Design review of the part built by this model. Coordinates are the model's own, in mm. Face numbers are marked on the shaded views. A direction names the side the tool comes from. Round coordinates to 2 decimals unless told otherwise and drop trailing zeros. Order: outer loops, then holes, each group sorted by start corner. A loop starts at its lowest first (then second) coordinate and runs counter-clockwise, first axis right, second up. Notation, with made-up numbers: M 13,82 L 28,82 A18 ccw 28,92 Z; hole C 13,42 d9. An arc over 180 degrees is marked long. Write each question's results on one line, items separated by ' | '. Start each with the question number.
Item 1: Take a section at C-C, the plane y = -16. Write out the cut boundary in (x, z).
Item 2: Clearance check with flat-ended pins moving along their axes: pin 1 (4 mm diameter, centred on x = 100, z = 2.5, fed in from +Y); pin 2 (1.9 mm diameter, centred on y = -26.5, z = 5.5, fed in from -X); pin 3 (5 mm diameter, centred on x = 10, y = -42, fed in from -Z); pin 4 (1.5 mm diameter, centred on x = 132, z = 11.5, fed in from -Y). State where each tip first meets the part, or that it passes through.
Item 3: Wall thickness on line 1 (Y direction, x = 50, z = 5.75); line 2 (Y direction, x = 124, z = 6.5); line 3 (Y direction, x = 124, z = 2.25): over which ranges is each line inside the solid? List them lowest first. Write a range as [from, to].
Item 4: Take a section at D-D, the plane x = 126.5. Write out the cut boundary in (y, z).
Item 5: Take a section at A-A, the plane x = 17. Write out the cut boundary in (y, z), plus the area to 3 significant figures.
Item 6: Take a section at B-B, the plane y = -25. Write out the cut boundary in (x, z), plus the area to 3 significant figures.
Item 7: Machinability: for the marked faces 1, 2 and 3, which of the approach directions +Z, -Z, +X, -X, +Y, -Y give a long, thin tool a straight path to every point of the face, cutting with its end or side? Answer none if there is none.
Item 8: The part is to be moulded in two halves that separate along Y. For the marked faces 4, 5 and 6, say which applies: +Y half, -Y half, draft (parallel to the pull), parting line (faces both ways), or undercut.
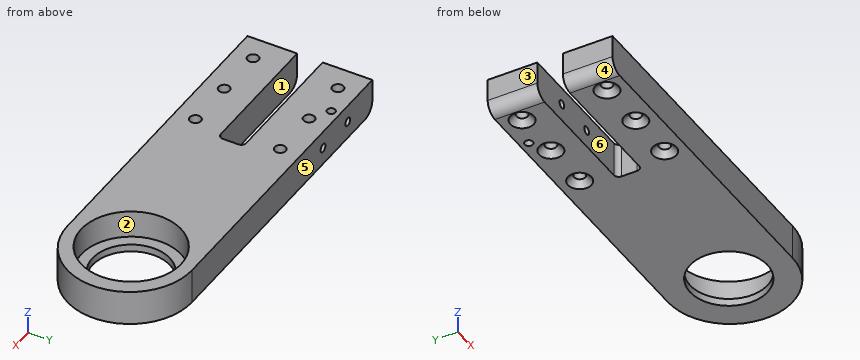
```python
from build123d import *

# Parameters (mm, degrees)
BOSS_EXTRUDE1_DEPTH       = 14
SKETCH2_W                 = 55
SKETCH2_H                 = 10.2
CUT_EXTRUDE1_DEPTH        = 15
F_8_CLEARANCE_HOLE1_D     = 4.5
F_8_CLEARANCE_HOLE1_DEPTH = 14
F_4_CLEARANCE_HOLE1_D     = 3.3
F_4_CLEARANCE_HOLE1_DEPTH = 14
F_4_CLEARANCE_HOLE2_D     = 3.3
F_4_CLEARANCE_HOLE2_DEPTH = 19.899999999
HOLE1_D                   = 31.000000009
HOLE1_DEPTH               = 14
HOLE1_CBORE_D             = 40.00000001
HOLE1_CBORE_DEPTH         = 11
CHAMFER1_SIZE             = 2.45
FILLET1_R                 = 2
FILLET2_R                 = 5


with BuildPart() as part:
    # Sketch1 → Boss-Extrude1 (new body)
    with BuildSketch(Plane(origin=(0, 0, 0), x_dir=(-1, 0, 0), z_dir=(0, 0, -1))):
        with BuildLine():
            Line((-125, -50), (0, -50))
            Line((0, -50), (0, 0))
            Line((0, 0), (-125, 0))
            ThreePointArc((-125, 0), (-150, -25), (-125, -50))
        make_face()
    extrude(amount=-BOSS_EXTRUDE1_DEPTH)

    # Sketch2 → Cut-Extrude1 (cut, through all)
    with BuildSketch(Plane.XY.offset(14)):
        with Locations((27.5, -24.999999999)):
            Rectangle(SKETCH2_W, SKETCH2_H)
    extrude(amount=-CUT_EXTRUDE1_DEPTH, mode=Mode.SUBTRACT)

    # #8 Clearance Hole1
    with Locations(Plane(origin=(0, 0, 0), x_dir=(-1, 0, 0), z_dir=(0, 0, -1))):
        with Locations((-10, -8), (-10, -42), (-30, -42), (-30, -8), (-50, -8), (-50, -42)):
            Hole(F_8_CLEARANCE_HOLE1_D / 2, depth=F_8_CLEARANCE_HOLE1_DEPTH)

    # #4 Clearance Hole1
    with Locations(Plane.XY.offset(14)):
        with Locations((22.5, -3.5)):
            Hole(F_4_CLEARANCE_HOLE1_D / 2, depth=F_4_CLEARANCE_HOLE1_DEPTH)

    # #4 Clearance Hole2
    with Locations(Plane(origin=(0, 0, 0), x_dir=(1, 0, 0), z_dir=(0, 1, 0))):
        with Locations((17, -7), (34.2, -7)):
            Hole(F_4_CLEARANCE_HOLE2_D / 2, depth=F_4_CLEARANCE_HOLE2_DEPTH)

    # Hole1
    with Locations(Plane.XY.offset(14)):
        with Locations((123.999999995, -24.999999999)):
            CounterBoreHole(HOLE1_D / 2, HOLE1_CBORE_D / 2, HOLE1_CBORE_DEPTH, depth=HOLE1_DEPTH)

    # Chamfer1
    chamfer1_edges = [part.edges().sort_by_distance(p)[0] for p in [
        (47.75, -42, 0),
        (47.75, -8, 0),
        (27.75, -8, 0),
        (27.75, -42, 0),
        (7.75, -42, 0),
        (7.75, -8, 0),
    ]]
    chamfer(chamfer1_edges, length=CHAMFER1_SIZE)

    # Fillet1
    fillet1_edges = [part.edges().sort_by_distance(p)[0] for p in [
        (55, -19.899999999, 7),
        (55, -30.099999999, 7),
    ]]
    fillet(fillet1_edges, radius=FILLET1_R)

    # Fillet2
    fillet2_edges = [part.edges().sort_by_distance(p)[0] for p in [
        (0, -9.95, 0),
        (0, -40.05, 0),
    ]]
    fillet(fillet2_edges, radius=FILLET2_R)


solid = part.part
```
Results list:
1) outline: M 0,5 A5 ccw 5,0 L 111.38,0 L 111.38,3 L 106.14,3 L 106.14,14 L 0,14 Z; M 136.62,0 L 148.32,0 L 148.32,14 L 141.86,14 L 141.86,3 L 136.62,3 Z; hole C 17,7 d3.3; hole C 34.2,7 d3.3
2) pin 1: y = 0 | pin 2: x = 55 | pin 3: z = 2.2 | pin 4: y = -49.21
3) line 1: [-50, -44.25], [-39.75, -30.1], [-19.9, -10.25], [-5.75, 0] | line 2: [-50, -45], [-5, 0] | line 3: [-50, -40.5], [-9.5, 0]
4) outline: M -49.95,0 L -40.3,0 L -40.3,3 L -44.84,3 L -44.84,14 L -49.95,14 Z; M -9.7,0 L -0.05,0 L -0.05,14 L -5.16,14 L -5.16,3 L -9.7,3 Z
5) outline: M -50,0 L -30.1,0 L -30.1,14 L -50,14 Z; M -19.9,0 L 0,0 L 0,5.35 L -19.9,5.35 Z; M -19.9,8.65 L 0,8.65 L 0,14 L -19.9,14 Z | area: 492 mm²
6) outline: M 55,0 L 108.5,0 L 108.5,3 L 104,3 L 104,14 L 55,14 Z; M 139.5,0 L 150,0 L 150,14 L 144,14 L 144,3 L 139.5,3 Z | area: 797 mm²
7) face 1: +Z, -Z, -X | face 2: +Z | face 3: +Z, -Z, -X, +Y, -Y
8) face 4: draft | face 5: +Y half | face 6: undercut
